Input: part model. Units: mm. Frame: model coordinates. A direction names the side the tool comes from. Coordinates: 2 decimals unless noted, no trailing zeros. Loops run counter-clockwise (first coordinate to the right, second up) from the corner with the lowest first, then second, coordinate; pieces in that order, holes last.
(1) Set-up query: faces 1 (the face through (7.395, 11.826, 47.61)), 2 (the face through (12.27, 1.5, 60.21)). Return all of +Z, -Z, +X, -X, +Y, -Y with unobstructed straight access to the full face (end or side cutting, diameter ignored); none if empty.
(2) Contact query for flat-ended pins moving along their axis: P1, Ø6, axis at x = 7, z = 18, coming from the -Y side; P2, Ø12, axis at y = 13.5, z = 20.5, coming from the -X side; P3, Ø4, axis at x = 5, z = -9, coming from the +Y side; P4, Ø3, axis at x = 8.5, y = 1, coming from the +Z side. Output: stop coordinate, or through.
(3) Section B-B, the plane y = 19. Return loops of the section in (x, z), then the cut area to 3 significant figures.
(4) Mould query, pull axis Y, two halves, no side actions, for faces 3 (the face through (0, 0, 13)), 4 (the face through (7, 0, 45)), 5 (the face through (7.395, -11.776, 48.366)). Classes: released by +Y, released by -Y, zero draft, split by the parting line, or undercut.
(5) Line query: L1, parallel to Z at x = 1.25, y = -5.5; L2, parallel to Z at x = 1, y = -4; L3, parallel to Y at x = 12, z = -4. Output: solid intervals per line, ascending.
(6) Section A-A, the plane z = 35. Return loops of the section in (x, y), then the cut area to 3 significant figures.
```python
from build123d import *

# Parameters (mm, degrees)
SKETCH1_R           = 6
BOSS_EXTRUDE1_DEPTH = 15
SKETCH2_R           = 5
CUT_EXTRUDE1_DEPTH  = 30
BOSS_EXTRUDE2_DEPTH = 15


with BuildPart() as part:
    # Sketch1 → Boss-Extrude1 (new body)
    with BuildSketch(Plane(origin=(0, 0, 0), x_dir=(0, 0, -1), z_dir=(1, 0, 0))):
        with BuildLine():
            ThreePointArc((25, 0), (7.092163634, 23.972926709), (-20.976097199, 13.60159352))
            ThreePointArc((-20.976097199, 13.60159352), (-25, 0), (-20.976097199, -13.60159352))
            ThreePointArc((-20.976097199, -13.60159352), (7.092163634, -23.972926709), (25, 0))
        make_face()
        Circle(SKETCH1_R, mode=Mode.SUBTRACT)
        with BuildLine():
            ThreePointArc((-20.976097199, -13.60159352), (-25, 0), (-20.976097199, 13.60159352))
            Line((-20.976097199, 13.60159352), (-75, 10))
            Line((-75, 10), (-75, -10))
            Line((-75, -10), (-20.976097199, -13.60159352))
        make_face()
    extrude(amount=BOSS_EXTRUDE1_DEPTH)

    # Sketch2 → Cut-Extrude1 (cut)
    with BuildSketch(Plane.XY.offset(75)):
        with Locations((7.5, 0)):
            Circle(SKETCH2_R)
    extrude(amount=-CUT_EXTRUDE1_DEPTH, mode=Mode.SUBTRACT)

    # Sketch4 → Boss-Extrude2 (add)
    with BuildSketch(Plane(origin=(15, 0, 0), x_dir=(0, 0, -1), z_dir=(1, 0, 0))):
        with BuildLine():
            Line((0.623259764, 4.490102446), (0.824935512, 5.943019552))
            ThreePointArc((0.824935512, 5.943019552), (1.24671071, 5.869046976), (1.662135778, 5.765180366))
            Line((1.662135778, 5.765180366), (1.25578586, 4.355740418))
            ThreePointArc((1.25578586, 4.355740418), (0.941921654, 4.434214283), (0.623259764, 4.490102446))
        make_face()
        with BuildLine():
            Line((1.863021407, 4.132629181), (2.465861922, 5.469874312))
            ThreePointArc((2.465861922, 5.469874312), (2.849711777, 5.280070339), (3.219046605, 5.063372291))
            Line((3.219046605, 5.063372291), (2.432071594, 3.825506564))
            ThreePointArc((2.432071594, 3.825506564), (2.153029737, 3.989227452), (1.863021407, 4.132629181))
        make_face()
        with BuildLine():
            Line((2.951852135, 3.440354878), (3.907018863, 4.553592384))
            ThreePointArc((3.907018863, 4.553592384), (4.221846144, 4.263333806), (4.515169421, 3.951359905))
            Line((4.515169421, 3.951359905), (3.411325351, 2.98535292))
            ThreePointArc((3.411325351, 2.98535292), (3.189712154, 3.221057138), (2.951852135, 3.440354878))
        make_face()
        with BuildLine():
            Line((3.801541359, 2.469363482), (5.031652372, 3.268405484))
            ThreePointArc((5.031652372, 3.268405484), (5.251951644, 2.901207322), (5.445500063, 2.51923184))
            Line((5.445500063, 2.51923184), (4.114213817, 1.903343737))
            ThreePointArc((4.114213817, 1.903343737), (3.967983063, 2.191935931), (3.801541359, 2.469363482))
        make_face()
        with BuildLine():
            Line((4.34325231, 1.298318944), (5.74865133, 1.718431809))
            ThreePointArc((5.74865133, 1.718431809), (5.856575257, 1.304042275), (5.934668676, 0.883010593))
            Line((5.934668676, 0.883010593), (4.483793147, 0.667136964))
            ThreePointArc((4.483793147, 0.667136964), (4.424791583, 0.98523711), (4.34325231, 1.298318944))
        make_face()
        with BuildLine():
            Line((4.53309879, 0.022092326), (5.999928747, 0.029241008))
            ThreePointArc((5.999928747, 0.029241008), (5.986733973, -0.398768521), (5.943045727, -0.82474692))
            Line((5.943045727, -0.82474692), (4.490122222, -0.623117278))
            ThreePointArc((4.490122222, -0.623117278), (4.523129803, -0.301279761), (4.53309879, 0.022092326))
        make_face()
        with BuildLine():
            Line((4.355700565, -1.255924081), (5.765127618, -1.662318725))
            ThreePointArc((5.765127618, -1.662318725), (5.631883107, -2.069273464), (5.469952559, -2.465688343))
            Line((5.469952559, -2.465688343), (4.132688299, -1.862890264))
            ThreePointArc((4.132688299, -1.862890264), (4.255030947, -1.563388739), (4.355700565, -1.255924081))
        make_face()
        with BuildLine():
            Line((3.825429385, -2.432192989), (5.063270137, -3.219207281))
            ThreePointArc((5.063270137, -3.219207281), (4.820770566, -3.572138177), (4.553716365, -3.906874361))
            Line((4.553716365, -3.906874361), (3.440448548, -2.95174296))
            ThreePointArc((3.440448548, -2.95174296), (3.64221479, -2.698841258), (3.825429385, -2.432192989))
        make_face()
        with BuildLine():
            Line((2.985244666, -3.411420085), (3.951216622, -4.515294808))
            ThreePointArc((3.951216622, -4.515294808), (3.619107863, -4.785609499), (3.268565153, -5.031548652))
            Line((3.268565153, -5.031548652), (2.469484116, -3.801462996))
            ThreePointArc((2.469484116, -3.801462996), (2.734328051, -3.615649709), (2.985244666, -3.411420085))
        make_face()
        with BuildLine():
            Line((1.903213179, -4.114274214), (2.519059035, -5.445580004))
            ThreePointArc((2.519059035, -5.445580004), (2.124246566, -5.6113792), (1.718614231, -5.748596796))
            Line((1.718614231, -5.748596796), (1.298456769, -4.343211108))
            ThreePointArc((1.298456769, -4.343211108), (1.604922315, -4.239539724), (1.903213179, -4.114274214))
        make_face()
        with BuildLine():
            Line((0.666994679, -4.483814315), (0.882822266, -5.934696694))
            ThreePointArc((0.882822266, -5.934696694), (0.457291444, -5.982548331), (0.029431406, -5.999927816))
            Line((0.029431406, -5.999927816), (0.022236176, -4.533098087))
            ThreePointArc((0.022236176, -4.533098087), (0.345495319, -4.519967444), (0.666994679, -4.483814315))
        make_face()
        with BuildLine():
            Line((-0.623259764, -4.490102446), (-0.824935512, -5.943019552))
            ThreePointArc((-0.824935512, -5.943019552), (-1.24671071, -5.869046976), (-1.662135778, -5.765180366))
            Line((-1.662135778, -5.765180366), (-1.25578586, -4.355740418))
            ThreePointArc((-1.25578586, -4.355740418), (-0.941921654, -4.434214283), (-0.623259764, -4.490102446))
        make_face()
        with BuildLine():
            Line((-1.863021407, -4.132629181), (-2.465861922, -5.469874312))
            ThreePointArc((-2.465861922, -5.469874312), (-2.849711777, -5.280070339), (-3.219046605, -5.063372291))
            Line((-3.219046605, -5.063372291), (-2.432071594, -3.825506564))
            ThreePointArc((-2.432071594, -3.825506564), (-2.153029737, -3.989227452), (-1.863021407, -4.132629181))
        make_face()
        with BuildLine():
            Line((-2.951852135, -3.440354878), (-3.907018863, -4.553592384))
            ThreePointArc((-3.907018863, -4.553592384), (-4.221846144, -4.263333806), (-4.515169421, -3.951359905))
            Line((-4.515169421, -3.951359905), (-3.411325351, -2.98535292))
            ThreePointArc((-3.411325351, -2.98535292), (-3.189712154, -3.221057138), (-2.951852135, -3.440354878))
        make_face()
        with BuildLine():
            Line((-3.801541359, -2.469363482), (-5.031652372, -3.268405484))
            ThreePointArc((-5.031652372, -3.268405484), (-5.251951644, -2.901207322), (-5.445500063, -2.51923184))
            Line((-5.445500063, -2.51923184), (-4.114213817, -1.903343737))
            ThreePointArc((-4.114213817, -1.903343737), (-3.967983063, -2.191935931), (-3.801541359, -2.469363482))
        make_face()
        with BuildLine():
            Line((-4.34325231, -1.298318944), (-5.74865133, -1.718431809))
            ThreePointArc((-5.74865133, -1.718431809), (-5.856575257, -1.304042275), (-5.934668676, -0.883010593))
            Line((-5.934668676, -0.883010593), (-4.483793147, -0.667136964))
            ThreePointArc((-4.483793147, -0.667136964), (-4.424791583, -0.98523711), (-4.34325231, -1.298318944))
        make_face()
        with BuildLine():
            Line((-4.53309879, -0.022092326), (-5.999928747, -0.029241008))
            ThreePointArc((-5.999928747, -0.029241008), (-5.986733973, 0.398768521), (-5.943045727, 0.82474692))
            Line((-5.943045727, 0.82474692), (-4.490122222, 0.623117278))
            ThreePointArc((-4.490122222, 0.623117278), (-4.523129803, 0.301279761), (-4.53309879, -0.022092326))
        make_face()
        with BuildLine():
            Line((-4.355700565, 1.255924081), (-5.765127618, 1.662318725))
            ThreePointArc((-5.765127618, 1.662318725), (-5.631883107, 2.069273464), (-5.469952559, 2.465688343))
            Line((-5.469952559, 2.465688343), (-4.132688299, 1.862890264))
            ThreePointArc((-4.132688299, 1.862890264), (-4.255030947, 1.563388739), (-4.355700565, 1.255924081))
        make_face()
        with BuildLine():
            Line((-3.825429385, 2.432192989), (-5.063270137, 3.219207281))
            ThreePointArc((-5.063270137, 3.219207281), (-4.820770566, 3.572138177), (-4.553716365, 3.906874361))
            Line((-4.553716365, 3.906874361), (-3.440448548, 2.95174296))
            ThreePointArc((-3.440448548, 2.95174296), (-3.64221479, 2.698841258), (-3.825429385, 2.432192989))
        make_face()
        with BuildLine():
            Line((-2.985244666, 3.411420085), (-3.951216622, 4.515294808))
            ThreePointArc((-3.951216622, 4.515294808), (-3.619107863, 4.785609499), (-3.268565153, 5.031548652))
            Line((-3.268565153, 5.031548652), (-2.469484116, 3.801462996))
            ThreePointArc((-2.469484116, 3.801462996), (-2.734328051, 3.615649709), (-2.985244666, 3.411420085))
        make_face()
        with BuildLine():
            Line((-1.903213179, 4.114274214), (-2.519059035, 5.445580004))
            ThreePointArc((-2.519059035, 5.445580004), (-2.124246566, 5.6113792), (-1.718614231, 5.748596796))
            Line((-1.718614231, 5.748596796), (-1.298456769, 4.343211108))
            ThreePointArc((-1.298456769, 4.343211108), (-1.604922315, 4.239539724), (-1.903213179, 4.114274214))
        make_face()
        with BuildLine():
            Line((-0.666994679, 4.483814315), (-0.882822266, 5.934696694))
            ThreePointArc((-0.882822266, 5.934696694), (-0.457291444, 5.982548331), (-0.029431406, 5.999927816))
            Line((-0.029431406, 5.999927816), (-0.022236176, 4.533098087))
            ThreePointArc((-0.022236176, 4.533098087), (-0.345495319, 4.519967444), (-0.666994679, 4.483814315))
        make_face()
    extrude(amount=-BOSS_EXTRUDE2_DEPTH)


solid = part.part
```
Report:
1. face 1: +Z, +X, -X, +Y
1. face 2: +Z
2. P1: stops at y = -20
2. P2: stops at x = 0
2. P3: stops at y = 24
2. P4: stops at z = 45
3. outline: (0, -16.25) - (15, -16.25) - (15, 16.25) - (0, 16.25) - close
3. area: 487 mm2
4. face 3: zero draft
4. face 4: undercut
4. face 5: released by -Y
5. L1: z = -24.39 to -1.64, -0.82 to -0.03, 0.76 to 1.59, 2.4 to 75
5. L2: z = -24.68 to -4.47, -3.5 to -2.6, 2.13 to 2.54, 3.43 to 75
5. L3: y = -24.68 to -4.47, -3.43 to -2.54, 2.13 to 2.6, 3.5 to 24.68
6. outline: (0, -12.67) - (15, -12.67) - (15, 12.67) - (0, 12.67) - close
6. area: 380 mm2
